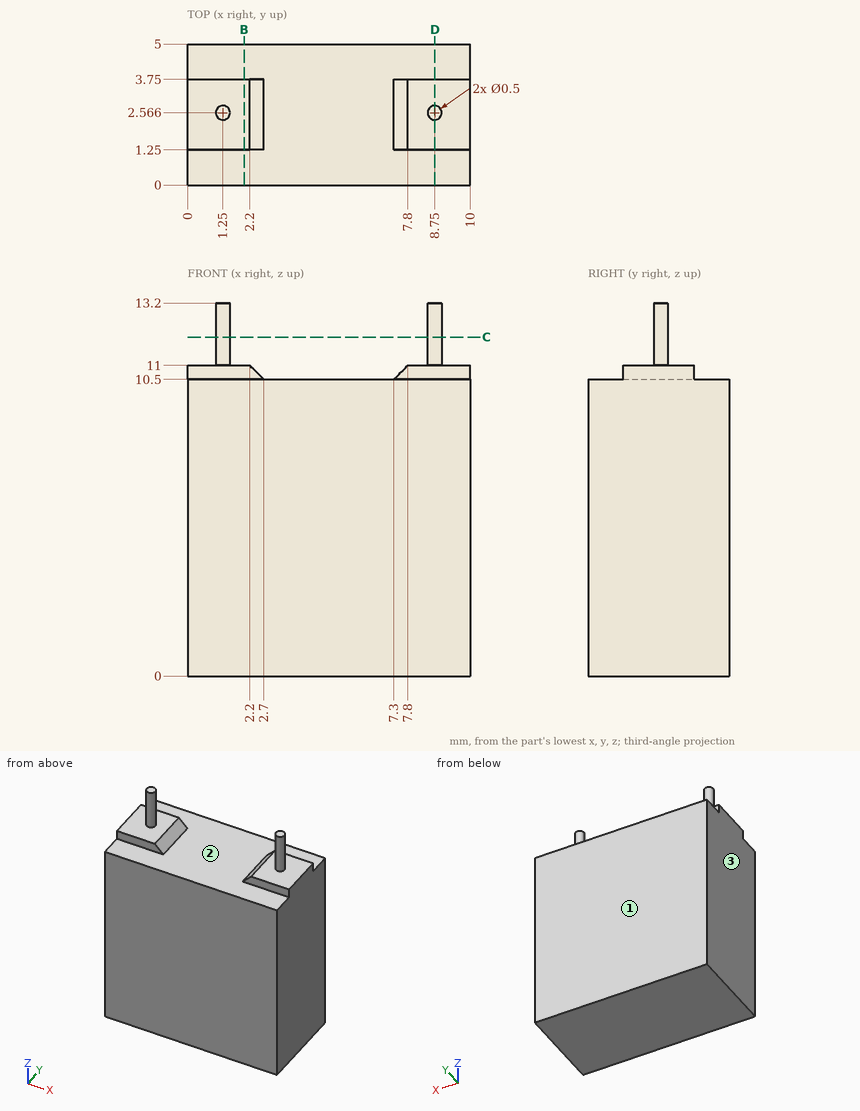
Design review of the part shown in the three views and the two pictorial views. Dimensions are in mm from the part's minimum x, y and z. Give positions to 0.01 mm unless a question says otherwise; leave off trailing zeros. Write each loop counter-clockwise with the first axis right and the second up, starting at its lowest first coordinate (ties: lowest second). Pieces come first, ordered by that corner, then holes. Notation, with made-up numbers: M -31,88 L 0,88 A18 ccw 0,100 Z; hole C -8.75,-16 d5. An arc over 180 degrees is marked long. One line per item, written item: value.
1) For P1, Ø2, axis at x = 3, y = 0.5, coming from the -Z side, flat-tipped, find the tip position at first contact; note if it passes through.
Results are:
P1: stops at z = 0
2) Take a section at D-D, the plane x = 8.75. Write out the cut boundary in (y, z).
Results are:
outline: M 0,0 L 5,0 L 5,10.5 L 3.75,10.5 L 3.75,11 L 2.82,11 L 2.82,13.2 L 2.32,13.2 L 2.32,11 L 1.25,11 L 1.25,10.5 L 0,10.5 Z
3) Take a section at C-C, the plane z = 12. Write out the cut boundary in (x, y).
Results are:
outline: C 1.25,2.57 d0.5; C 8.75,2.57 d0.5
4) The part is to be moulded in two halves that separate along X. For the marked faces 1, 2 and 3, say which applies: +X half, -X half, draft (parallel to the pull), parting line (faces both ways), or undercut.
Results are:
face 1: draft
face 2: undercut
face 3: -X half
5) For line 1 (Z direction, x = 2, y = 0.9); line 2 (Z direction, x = 9, y = 1.4); line 3 (X direction, y = 2.8, z = 10.75), list the stretches that pass through material, from the lowest coordinate up. Write a range as from..to.
Results are:
line 1: z = 0..10.5
line 2: z = 0..11
line 3: x = 0..2.45, 7.55..10
6) Take a section at B-B, the plane x = 2. Write out the cut boundary in (y, z).
Results are:
outline: M 0,0 L 5,0 L 5,10.5 L 3.75,10.5 L 3.75,11 L 1.25,11 L 1.25,10.5 L 0,10.5 Z
